```python
from build123d import *

# Parameters (mm, degrees)
F0_R     = 9.525
F0_R_2   = 6.4135
F1_DEPTH = 2.794
F2_SIZE  = 0.508


with BuildPart() as f1:
    # F0 (on Right) → F1 (new body)
    with BuildSketch(Plane.YZ):
        Circle(F0_R)
        Circle(F0_R_2, mode=Mode.SUBTRACT)
    extrude(amount=F1_DEPTH)

    # F2
    f2_edges = [f1.edges().sort_by_distance(p)[0] for p in [
        (1.397, 6.4135, 0),
        (0, -6.4135, 0),
        (2.794, -6.4135, 0),
        (1.397, 9.525, 0),
        (0, -9.525, 0),
        (2.794, -9.525, 0),
    ]]
    chamfer(f2_edges, length=F2_SIZE)


solid = f1.part
```
The listing builds one solid part. Answer for the finished solid, in the listing's coordinates (mm). Round coordinates to 2 decimals unless told otherwise and drop trailing zeros. Write each loop counter-clockwise with the first axis right and the second up, starting at its lowest first coordinate (ties: lowest second). Pieces come first, ordered by that corner, then holes. Notation, with made-up numbers: (88.25, 53.25) -> (107.25, 53.25) arc R37 cw to (107.25, 92.25) -> close; hole circle Ø7 at (74, -37.75). An arc over 180 degrees is marked (long way). Use CSV: the item, a comma, the result in double quotes. Start each with the question number.
(1) The mould has two halves that part along Z. Classify faces 1 (the face through (0, -2, -7)), 2 (the face through (1.385, 6.117, 1.926)), 3 (the face through (1.385, -7.559, -5.796)): released by +Z, released by -Z, zero draft, split by the parting line, or undercut.
(2) Section A-A on z = 0 is taken. Give the vertices of the cut face in (x, y) (1 decimal).
(3) Consider L1, parallel to Z at x = 1.5, y = 0 (1 decimal); L2, parallel to Y at x = 2.35, z = 0.5; L3, parallel to Z at x = 2.3, y = -2.75. Determine where each line is inside the solid, lowest interval first. Write a range as from..to.
(4) This flat-tipped pin is pushed along its axis until it touches: pin 1 (1 mm diameter, centred on x = 0.5, y = 0.5, fed in from +Z) (3 decimals). Where does it stop, or does it pass through?
A:
1,face 1,"zero draft"
1,face 2,"undercut"
1,face 3,"split by the parting line"
2,outline,"(0, -9) -> (0.5, -9.5) -> (2.3, -9.5) -> (2.8, -9) -> (2.8, -6.9) -> (2.3, -6.4) -> (0.5, -6.4) -> (0, -6.9) -> close; (0, 6.9) -> (0.5, 6.4) -> (2.3, 6.4) -> (2.8, 6.9) -> (2.8, 9) -> (2.3, 9.5) -> (0.5, 9.5) -> (0, 9) -> close"
3,L1,"z = -9.5..-6.4, 6.4..9.5"
3,L2,"y = -9.45..-6.46, 6.46..9.45"
3,L3,"z = -9.1..-5.81, 5.81..9.1"
4,pin 1,"stops at z = 9.525"
